from build123d import *

# Parameters (mm, degrees)
BOSS_EXTRUDE1_DEPTH = 100
CIRPATTERN1_COUNT   = 4


# Read off the part's stored shape, not the designer's step: M5 Tapped Hole1
with BuildPart() as part:
    # Sketch1 → Boss-Extrude1 (new, symmetric)
    with BuildSketch(Plane(origin=(0, 0, 0), x_dir=(0, 0, -1), z_dir=(1, 0, 0))):
        with BuildLine():
            Line((0, 2), (0, 3.7))
            Line((0, 3.7), (-0.2, 3.9))
            Line((-0.2, 3.9), (-2.839339827, 3.9))
            Line((-2.839339827, 3.9), (-5.5, 6.560660173))
            Line((-5.5, 6.560660173), (-5.5, 8.2))
            Line((-5.5, 8.2), (-3.262842712, 8.2))
            ThreePointArc((-3.262842712, 8.2), (-3.078066806, 8.323463314), (-3.121421356, 8.541421356))
            Line((-3.121421356, 8.541421356), (-4.401335137, 9.821335137))
            ThreePointArc((-4.401335137, 9.821335137), (-4.599233379, 9.953566515), (-4.832670273, 10))
            Line((-4.832670273, 10), (-9.5, 10))
            ThreePointArc((-9.5, 10), (-9.853553391, 9.853553391), (-10, 9.5))
            Line((-10, 9.5), (-10, 4.832670273))
            ThreePointArc((-10, 4.832670273), (-9.953566515, 4.599233379), (-9.821335137, 4.401335137))
            Line((-9.821335137, 4.401335137), (-8.541421356, 3.121421356))
            ThreePointArc((-8.541421356, 3.121421356), (-8.323463314, 3.078066806), (-8.2, 3.262842712))
            Line((-8.2, 3.262842712), (-8.2, 5.5))
            Line((-8.2, 5.5), (-6.560660173, 5.5))
            Line((-6.560660173, 5.5), (-3.9, 2.839339827))
            Line((-3.9, 2.839339827), (-3.9, 0.2))
            Line((-3.9, 0.2), (-3.7, 0))
            Line((-3.7, 0), (-2, 0))
            ThreePointArc((-2, 0), (-1.414213562, 1.414213562), (0, 2))
        make_face()
    boss_extrude1 = extrude(amount=BOSS_EXTRUDE1_DEPTH, both=True)

    # CirPattern1: Boss-Extrude1 ×4 about axis
    cirpattern1_axis = Axis((0, 0, 0), (1, 0, 0))
    for i in range(1, CIRPATTERN1_COUNT):
        add(boss_extrude1.rotate(cirpattern1_axis, i * 360 / CIRPATTERN1_COUNT))

    # M5 Tapped Hole1 outline → M5 Tapped Hole1 (revolve, cut)
    with BuildSketch(Plane.YX):
        Polygon((2.1, -87.6), (2, -87.539913938), (2, -100), (2.1, -100), align=None)
        Polygon((2, 100), (2, 87.539913938), (2.1, 87.6), (2.1, 100), align=None)
    revolve(axis=Axis((0, 0, 0), (1, 0, 0)), mode=Mode.SUBTRACT)


solid = part.part
CAD build for the part. Positions are in the model's coordinates, mm. Round coordinates to 2 decimals unless told otherwise and drop trailing zeros.
(1) Probe line 1 along Y through (x, z) = (8.5, 7); line 2 along Z through (x, y) = (-82.5, -3.25). List the from-to ranges inside material, lowest first.
(2) Mould opens along Y. For faces 1 (the face through (1, 10, -7)), 2 (the face through (1, -10, -7)), 3 (the face through (93.887, 2.003, 0.631)) say: pulls with the +Y half, pulls with the -Y half, needs draft (parallel to the pull), parting line crosses it, or undercut.
(3) Drop flat-ended pins along their axis: P1, Ø1.1, axis at x = 25, y = 4, coming from the +Z side; P2, Ø3, axis at x = 47, y = -1, coming from the +Z side; P3, Ø0.7, axis at x = 27, y = -4, coming from the -Z side. Give the stop position or say it passes through.
From the geometry:
1. line 1: y = -10 to -5.5, 5.5 to 10
1. line 2: z = -8.67 to -8.2, -4.31 to 4.31, 8.2 to 8.67
2. face 1: pulls with the +Y half
2. face 2: pulls with the -Y half
2. face 3: undercut
3. P1: stops at z = 9.93
3. P2: stops at z = 3.9
3. P3: stops at z = -9.77
